Here's how the part is built. I have some questions about the finished solid (model axes, mm). A direction names the side the tool comes from. Give positions to 0.01 mm unless a question says otherwise; leave off trailing zeros. Write each loop counter-clockwise with the first axis right and the second up, starting at its lowest first coordinate (ties: lowest second). Pieces come first, ordered by that corner, then holes. Notation, with made-up numbers: (16.25, -19) - (57.25, -19) arc R22 cw to (57.25, 3) - close; hole circle Ø3 at (-11.5, 82). An arc over 180 degrees is marked (long way). One line per item, written item: value. Start each with the question number.
1) Imagine slicing it at C-C on z = -19.5. Write out the boundary of the cut face in (x, y), plus the area to 3 significant figures.
2) I'm going to push flat-ended pins straight in: P1, Ø3, axis at y = 1, z = -3.5, coming from the -X side; P2, Ø2.5, axis at x = 21, y = 3.5, coming from the -Z side; P3, Ø3, axis at x = 65, y = 3, coming from the -Z side. Where does each tip first touch, or does it pass through?
3) Please list where these lines run through material, in increasing order: L1, parallel to X at y = 1.1, z = 0; L2, parallel to X at y = 3.55, z = 1; L3, parallel to Z at x = 43, y = 4.65. Write a range as [from, to].
4) On a 3-axis mill with a long thin cutter (end or side, diameter ignored), from which of +Z, -Z, +X, -X, +Y, -Y can I reach the whole of each face in a straight line? I mean faces 4 (the flat face through (23, 2, -12)), 5 (the cylindrical face through (-3.905, 2.465, -0.867)), 6 (the flat face through (81.743, 2.465, -4.197)). Say none if no direction works.
5) We'd pull the mould along X, two halves only. Please class faces 1 (the flat face through (123.123, 2.465, -8.194)), 2 (the cylindrical face through (46.095, 2.465, -0.867)), 3 (the flat face through (73.093, 2.465, -17.693)): +X half, -X half, draft (parallel to the pull), parting line (faces both ways), or undercut.
6) Imagine slicing it at B-B on x = 8. Write out the boundary of the cut face in (y, z).
7) Imagine slicing it at A-A on y = 1.15. Write out the boundary of the cut face in (x, z), plus the area to 3 significant figures.
from build123d import *

# Parameters (mm, degrees)
SKETCH1_R           = 4
BOSS_EXTRUDE1_DEPTH = 5
FILLET1_R           = 5


with BuildPart() as part:
    # Sketch1 → Boss-Extrude1 (new body)
    with BuildSketch(Plane(origin=(0, 0, 0), x_dir=(1, 0, 0), z_dir=(0, 1, 0))):
        with BuildLine():
            Line((0, 12), (46.309546143, 12))
            Line((46.309546143, 12), (100.107664183, 23.435142995))
            ThreePointArc((100.107664183, 23.435142995), (113.686830565, 20.974303457), (122.439553034, 10.304751439))
            Line((122.439553034, 10.304751439), (123.826560512, 6.023839123))
            Line((123.826560512, 6.023839123), (104.157567187, 1.843065531))
            Line((104.157567187, 1.843065531), (102, 8.502262467))
            Line((102, 8.502262467), (62, 0))
            ThreePointArc((62, 0), (58.485281374, -8.485281374), (50, -12))
            Line((50, -12), (0, -12))
            ThreePointArc((0, -12), (-12, 0), (0, 12))
        make_face()
        with Locations(Location((0, 0, 0), (0, 0, 270))):
            Circle(SKETCH1_R, mode=Mode.SUBTRACT)
        with Locations(Location((50, 0, 0), (0, 0, 270))):
            Circle(SKETCH1_R, mode=Mode.SUBTRACT)
    extrude(amount=BOSS_EXTRUDE1_DEPTH)

    # Fillet1
    fillet1_edges = [part.edges().sort_by_distance(p)[0] for p in [
        (102, 2.5, -8.502262467),
        (62, 2.5, 0),
        (46.309546143, 2.5, -12),
    ]]
    fillet(fillet1_edges, radius=FILLET1_R)


solid = part.part
Numbers:
1. outline: (81.59, 0) - (115.86, 0) - (115.86, 5) - (81.59, 5) - close
1. area: 171 mm^2
2. P1: x = -11.83
2. P2: z = -12
2. P3: z = -16.29
3. L1: [-12, -4], [4, 46], [54, 63.71]
3. L2: [-11.96, -3.87], [3.87, 46.13], [53.87, 62.61]
3. L3: [-12, 12]
4. face 4: -Z, -X, +Y, -Y
4. face 5: +Y, -Y
4. face 6: +Z, +Y, -Y
5. face 1: +X half
5. face 2: undercut
5. face 3: -X half
6. outline: (0, -12) - (5, -12) - (5, 12) - (0, 12) - close
7. outline: (0, -12) - (45.78, -12) arc R5 cw to (46.82, -12.11) - (100.11, -23.44) arc R20 ccw to (122.44, -10.3) - (123.83, -6.02) - (104.16, -1.84) - (103.39, -4.22) arc R5 cw to (97.59, -7.57) - (65.44, -0.73) arc R5 cw to (61.64, 2.94) arc R12 ccw to (50, 12) - (0, 12) arc R12 ccw to start; hole circle Ø8 at (0, 0); hole circle Ø8 at (50, 0)
7. area: 2,570 mm^2
